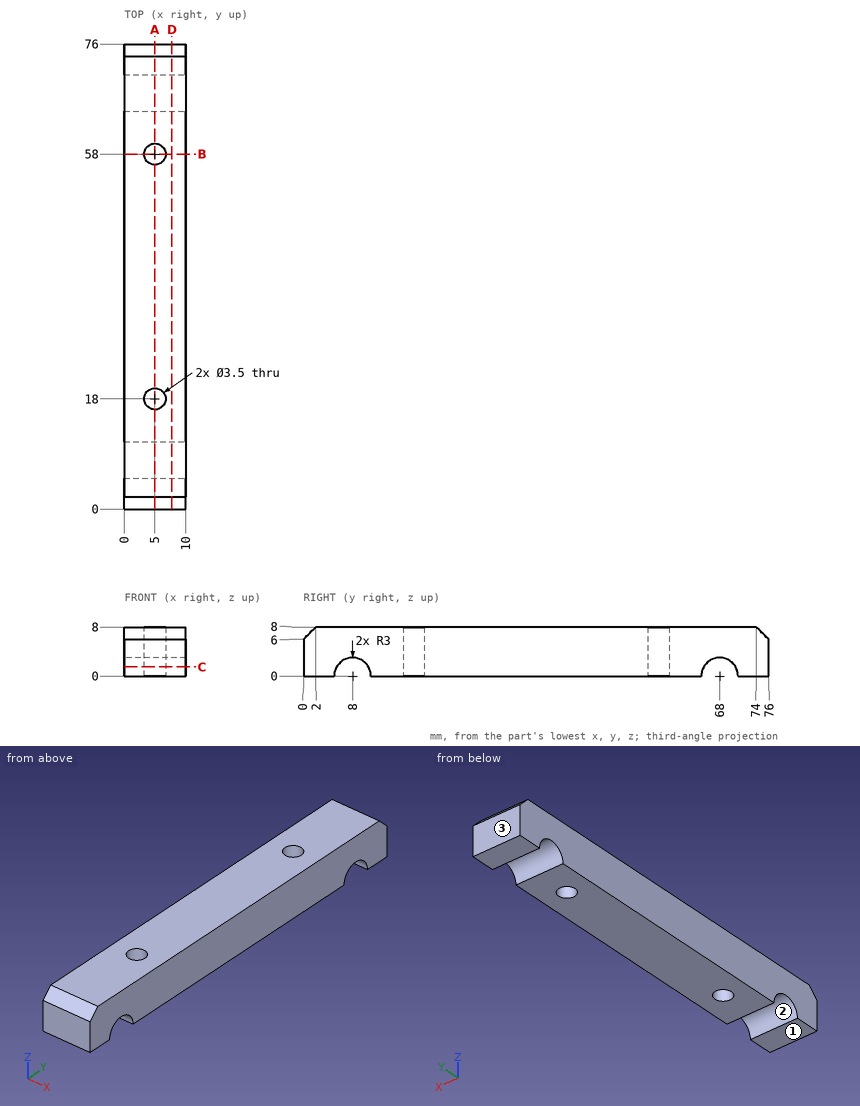
Study the drawing (mm; zero at the part's minimum x, y, z) and answer. Give positions to 0.01 mm unless a question says otherwise; leave off trailing zeros. Write each loop counter-clockwise with the first axis right and the second up, starting at its lowest first coordinate (ties: lowest second). Pieces come first, ordered by that corner, then holes. Notation, with made-up numbers: M 32.25,-35 L 65.25,-35 A22 cw 65.25,-26 Z; hole C 8,-0.5 d11. An arc over 180 degrees is marked long. Put each result on its own line as item: value. Start each with the question number.
1. The part is cut by section A-A, the plane x = 5. Give the vertices of the cut face in (y, z), and give its area (3 significant figures).
2. The part is cut by section C-C, the plane z = 1.5. Give the vertices of the cut face in (x, y).
3. For a pull along Y with two mould halves and no side action, classify the marked faces 1, 2 and 3 as released by +Y, released by -Y, zero draft, split by the parting line, or undercut.
4. The part is cut by section D-D, the plane x = 7.75. Give the vertices of the cut face in (y, z).
5. Consider line 1 along Y through (x, z) = (5, 6); line 2 along Y through (x, z) = (5, 6.25); line 3 along Y through (x, z) = (6.25, 2.25). Determine where each line is inside the solid, lowest interval first.
6. The part is cut by section B-B, the plane y = 58. Give the vertices of the cut face in (x, z).
Final values:
1. outline: M 0,0 L 5,0 A3 cw 11,0 L 16.25,0 L 16.25,8 L 2,8 L 0,6 Z; M 19.75,0 L 56.25,0 L 56.25,8 L 19.75,8 Z; M 59.75,0 L 65,0 A3 cw 71,0 L 76,0 L 76,6 L 74,8 L 59.75,8 Z
1. area: 520 mm²
2. outline: M 0,0 L 10,0 L 10,5.4 L 0,5.4 Z; M 0,10.6 L 10,10.6 L 10,65.4 L 0,65.4 Z; M 0,70.6 L 10,70.6 L 10,76 L 0,76 Z; hole C 5,18 d3.5; hole C 5,58 d3.5
3. face 1: zero draft
3. face 2: undercut
3. face 3: released by +Y
4. outline: M 0,0 L 5,0 A3 cw 11,0 L 65,0 A3 cw 71,0 L 76,0 L 76,6 L 74,8 L 2,8 L 0,6 Z
5. line 1: y = 0 to 16.25, 19.75 to 56.25, 59.75 to 76
5. line 2: y = 0.25 to 16.25, 19.75 to 56.25, 59.75 to 75.75
5. line 3: y = 0 to 6.02, 9.98 to 16.78, 19.22 to 56.78, 59.22 to 66.02, 69.98 to 76
6. outline: M 0,0 L 3.25,0 L 3.25,8 L 0,8 Z; M 6.75,0 L 10,0 L 10,8 L 6.75,8 Z
